```python
from build123d import *

# Parameters (mm, degrees)
EXTRUDE1_DEPTH     = 3.175
CUT_EXTRUDE2_DEPTH = 4.175
FILLET1_R          = 2.5
FILLET2_R          = 3.175


with BuildPart() as part:
    # Sketch1 → Extrude1 (new body)
    with BuildSketch(Plane(origin=(0, 0, 0), x_dir=(1, 0, 0), z_dir=(0, 1, 0))):
        Polygon((-69.865, 256.29975), (11.135, 256.29975), (11.135, 248.06225), (11.135, 238.53725), (11.135, 230.29975), (-27.865, 230.29975), (-27.865, -127.70025), (11.135, -127.70025), (11.135, -145.46275), (11.135, -153.70025), (-69.865, -153.70025), align=None)
        with BuildLine():
            Line((-8, -135.93775), (2, -135.93775))
            ThreePointArc((2, -135.93775), (6.7625, -140.70025), (2, -145.46275))
            Line((2, -145.46275), (-8, -145.46275))
            ThreePointArc((-8, -145.46275), (-12.7625, -140.70025), (-8, -135.93775))
        make_face(mode=Mode.SUBTRACT)
        with BuildLine():
            Line((-8, 248.06225), (2, 248.06225))
            ThreePointArc((2, 248.06225), (6.7625, 243.29975), (2, 238.53725))
            Line((2, 238.53725), (-8, 238.53725))
            ThreePointArc((-8, 238.53725), (-12.7625, 243.29975), (-8, 248.06225))
        make_face(mode=Mode.SUBTRACT)
    extrude(amount=EXTRUDE1_DEPTH)

    # Sketch2 → Cut-Extrude2 (cut, through all)
    with BuildSketch(Plane(origin=(0, 3.175, 0), x_dir=(1, 0, 0), z_dir=(0, 1, 0))):
        with BuildLine():
            Line((-0.2375, -135.93775), (-0.2375, -130.70025))
            Line((-0.2375, -130.70025), (6.7625, -130.70025))
            Line((6.7625, -130.70025), (6.7625, -140.70025))
            ThreePointArc((6.7625, -140.70025), (5.367596045, -137.332653955), (2, -135.93775))
            Line((2, -135.93775), (-0.2375, -135.93775))
        make_face()
    extrude(amount=-CUT_EXTRUDE2_DEPTH, mode=Mode.SUBTRACT)

    # Fillet1
    fillet1_edges = [part.edges().sort_by_distance(p)[0] for p in [
        (-0.2375, 1.5875, 135.93775),
        (-0.2375, 1.5875, 130.70025),
        (6.7625, 1.5875, 130.70025),
    ]]
    fillet(fillet1_edges, radius=FILLET1_R)

    # Fillet2
    fillet2_edges = [part.edges().sort_by_distance(p)[0] for p in [
        (-27.865, 1.5875, -230.29975),
        (-27.865, 1.5875, 127.70025),
    ]]
    fillet(fillet2_edges, radius=FILLET2_R)


solid = part.part
```
Read the model definition and answer for the solid it produces. Units are mm, in the model's axes. Give positions to 0.01 mm unless a question says otherwise; leave off trailing zeros. Write each loop counter-clockwise with the first axis right and the second up, starting at its lowest first coordinate (ties: lowest second). Pieces come first, ordered by that corner, then holes. Notation, with made-up numbers: (1.5, 0) -> (25.5, 0) arc R17 cw to (25.5, 17) -> close; hole circle Ø1 at (55.25, 11). An arc over 180 degrees is marked (long way). Answer in a Markdown table with one row per item.
1) Straight lines are drawn through the part: line 1 (Z direction, x = 1.5, y = 2.25); line 2 (Z direction, x = -23, y = 1.1); line 3 (Z direction, x = 0.5, y = 0.6). For each, find the intervals that lie inside material, in ascending order. Write a range as [from, to].
Results list:
| item | result |
|---|---|
| line 1 | [-256.3, -248.06], [-238.54, -230.3], [127.7, 130.82], [145.46, 153.7] |
| line 2 | [-256.3, -230.3], [127.7, 153.7] |
| line 3 | [-256.3, -248.06], [-238.54, -230.3], [127.7, 131.43], [145.46, 153.7] |
2) Section C-C on z = 67 is taken. Give the vertices of the cut face in (x, y) (3 decimals), plus the area to 3 significant figures.
Results list:
| item | result |
|---|---|
| outline | (-69.865, 0) -> (-27.865, 0) -> (-27.865, 3.175) -> (-69.865, 3.175) -> close |
| area | 133 mm^2 |
3) Section A-A on x = -18.5 is taken. Give the vertices of the cut face in (y, z) (3 decimals), plus the area to 3 significant figures.
Results list:
| item | result |
|---|---|
| outline | (0, -256.3) -> (3.175, -256.3) -> (3.175, -230.3) -> (0, -230.3) -> close; (0, 127.7) -> (3.175, 127.7) -> (3.175, 153.7) -> (0, 153.7) -> close |
| area | 165 mm^2 |
4) Section B-B on y = 1.7 is taken. Count the separate pieces of the cut face and the enclosed holes in it, plus the area to 3 significant figures.
Results list:
| item | result |
|---|---|
| separate pieces | 1 |
| enclosed holes | 2 |
| area | 18,900 mm^2 |
